Source: three-view drawing plus pictorial views. Frame: mm from the lowest corner of the part. Round coordinates to 2 decimals unless told otherwise and drop trailing zeros. Loops run counter-clockwise (first coordinate to the right, second up) from the corner with the lowest first, then second, coordinate; pieces in that order, holes last. Notation, with made-up numbers: (22, -5.5) -> (65, -5.5) arc R14 ccw to (65, -1.5) -> close; hole circle Ø10 at (34, 69). An arc over 180 degrees is marked (long way). Answer in a Markdown table with one row per item. Add a question column.
Q1. Section A-A, the plane z = 42.5. Output: boundary loops of the cut face in (x, y).
Q2. Ray query, L1, parallel to X at y = 0.85, z = 52.5 (1 decimal); L2, parallel to X at y = 3.2, z = 38 (1 decimal); L3, parallel to Z at x = 31.5, y = 2. Return the intervals inside material, ascending. Write a range as from..to.
Q3. Pin query (flat end, axial travel): pin 1 (1.5 mm diameter, centred on x = 10.5, y = 2.5, fed in from -Z). Return the tip coordinate at first contact, or that it passes through.
Q4. Section C-C, the plane z = 63.5. Output: boundary loops of the cut face in (x, y).
Q5. Section B-B, the plane y = 0.85. Give the number of separate pieces and of enclosed holes in the cut face, and give its area (3 significant figures).
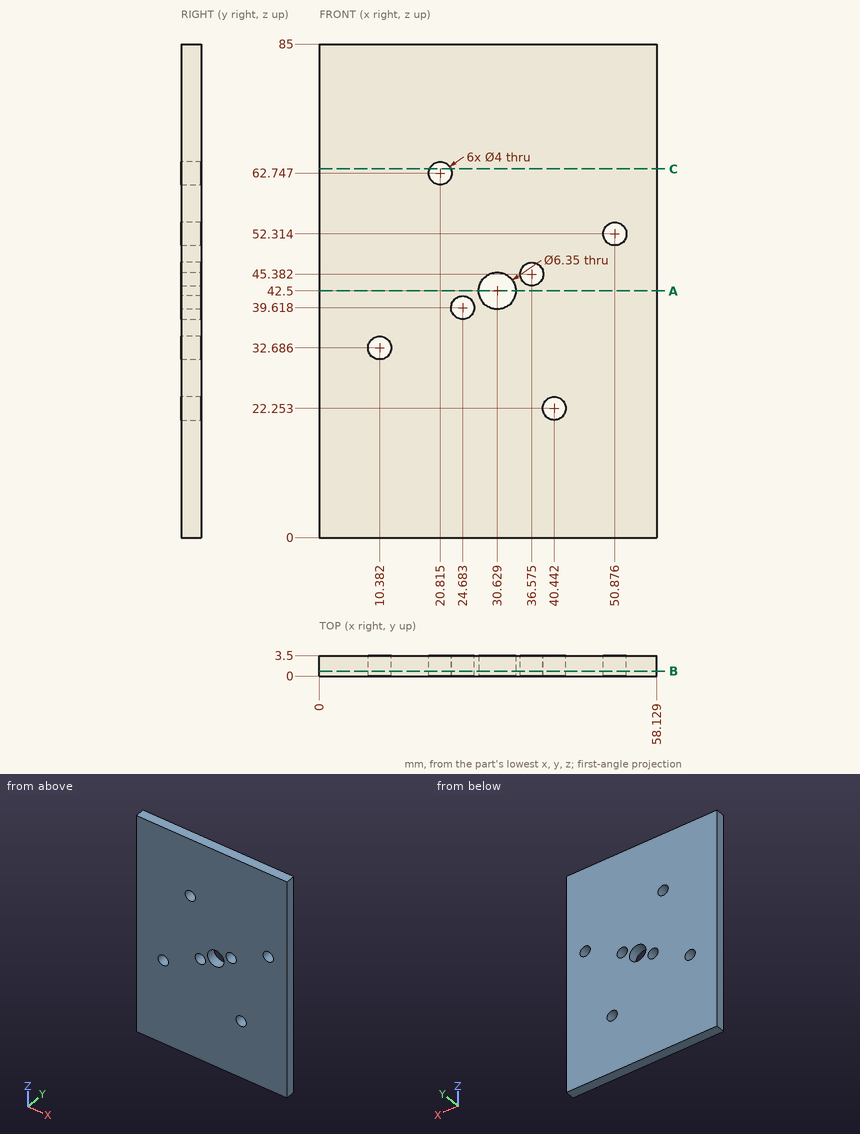
Answer block:
| question | item | result |
|---|---|---|
| 1 | outline | (0, 0) -> (27.45, 0) -> (27.45, 3.5) -> (0, 3.5) -> close; (33.8, 0) -> (58.13, 0) -> (58.13, 3.5) -> (33.8, 3.5) -> close |
| 2 | L1 | 0..48.9, 52.9..58.1 |
| 2 | L2 | 0..23.5, 25.9..58.1 |
| 2 | L3 | 0..39.45, 45.55..85 |
| 3 | pin 1 | z = 0 |
| 4 | outline | (0, 0) -> (18.96, 0) -> (18.96, 3.5) -> (0, 3.5) -> close; (22.67, 0) -> (58.13, 0) -> (58.13, 3.5) -> (22.67, 3.5) -> close |
| 5 | separate pieces | 1 |
| 5 | enclosed holes | 7 |
| 5 | area | 4,830 mm^2 |
